CAD build for the part. Positions are in the model's coordinates, mm. A direction names the side the tool comes from. Coordinates: 2 decimals unless noted, no trailing zeros. Loops run counter-clockwise (first coordinate to the right, second up) from the corner with the lowest first, then second, coordinate; pieces in that order, holes last.
1) Wall check: line 1 along Y through (x, z) = (35, -3.05); line 2 along Y through (x, z) = (3.15, -13); line 3 along Y through (x, z) = (44.2, -2.4). Give the ranges that are in metal, low to high.
2) Saw through at D-D, the plane z = -21. Write the cut outline in (x, y).
3) Two-plate mould, pull along Y, no slides. Class faces 3 (the flat face through (14, 0, -7)), 4 (the flat face through (0, 20, -14)), 5 (the cylindrical face through (3, 22, -21)): +Y half, -Y half, draft (parallel to the pull), parting line (faces both ways), or undercut.
4) Saw through at B-B, the plane y = 17. Write the cut outline in (x, z).
5) Saw through at A-A, the plane z = -13. Write the cut outline in (x, y).
6) Pin check, flat tips, straight feed: pin 1 Ø3.5 at (x, y) = (25.8, 8) entering from +Z; pin 2 Ø3 at (x, y) = (42.5, 9.5) entering from -Z. Stop position of each tip, or through.
7) Saw through at C-C, the plane x = 44.2. Write the cut outline in (y, z).
8) Which spindle directions (+Z, -Z, +X, -X, +Y, -Y) get a long thin tool onto all of the face, cutting with end or side? Do faces 1 (the flat face through (9, 35, -9)), 2 (the cylindrical face through (30.24, 24.35, -2.46)). Say none if no direction does.
```python
from build123d import *

# Parameters (mm, degrees)
BOSS_EXTRUDE1_DEPTH = 40
CUT_EXTRUDE1_DEPTH  = 35
BOSS_EXTRUDE2_DEPTH = 5
SKETCH6_R           = 2
CUT_EXTRUDE2_DEPTH  = 70.641941386
SKETCH7_R           = 3.2
SKETCH7_R_2         = 2.1
SKETCH7_R_3         = 2
CUT_EXTRUDE4_DEPTH  = 18.4
SKETCH9_R           = 5.05
CUT_EXTRUDE5_DEPTH  = 3
SKETCH10_R          = 6
CUT_EXTRUDE6_DEPTH  = 73.972597597
SKETCH11_W          = 8
SKETCH11_H          = 40
CUT_EXTRUDE7_DEPTH  = 70.641941386


with BuildPart() as part:
    # Sketch1 → Boss-Extrude1 (new body)
    with BuildSketch(Plane(origin=(0, 0, 0), x_dir=(1, 0, 0), z_dir=(0, 1, 0))):
        Polygon((0, 0), (50, 0), (50, 5), (20, 5), (5, 20), (5, 35), (0, 35), align=None)
    extrude(amount=BOSS_EXTRUDE1_DEPTH)

    # Sketch3 → Cut-Extrude1 (cut)
    with BuildSketch(Plane.XZ):
        Polygon((5, -20), (5, -5), (20, -5), align=None)
    extrude(amount=-CUT_EXTRUDE1_DEPTH, mode=Mode.SUBTRACT)

    # Sketch5 → Boss-Extrude2 (add)
    with BuildSketch(Plane.XZ):
        Polygon((5, -20), (5, -5), (20, -5), align=None)
    extrude(amount=-BOSS_EXTRUDE2_DEPTH)

    # Sketch6 → Cut-Extrude2 (cut, through all)
    with BuildSketch(Plane(origin=(5, 0, 0), x_dir=(0, 0, -1), z_dir=(1, 0, 0))):
        with Locations((13, 30)):
            Circle(SKETCH6_R)
        with Locations((13, 10)):
            Circle(SKETCH6_R)
        with Locations((21, 20)):
            Circle(SKETCH6_R)
    extrude(amount=-CUT_EXTRUDE2_DEPTH, mode=Mode.SUBTRACT)

    # Sketch7 → Cut-Extrude4 (cut)
    with BuildSketch(Plane(origin=(0, 0, -5), x_dir=(-1, 0, 0), z_dir=(0, 0, -1))):
        with Locations((-35, 28)):
            Circle(SKETCH7_R)
        with Locations((-35, 17)):
            Circle(SKETCH7_R_2)
        with Locations((-25.8, 8)):
            Circle(SKETCH7_R_3)
        with Locations((-44.2, 8)):
            Circle(SKETCH7_R_3)
    extrude(amount=-CUT_EXTRUDE4_DEPTH, mode=Mode.SUBTRACT)

    # Sketch9 → Cut-Extrude5 (cut)
    with BuildSketch(Plane.XY):
        with Locations((35, 28)):
            Circle(SKETCH9_R)
    extrude(amount=-CUT_EXTRUDE5_DEPTH, mode=Mode.SUBTRACT)

    # Sketch10 → Cut-Extrude6 (cut, through all)
    with BuildSketch(Plane.XY):
        with Locations((35, 28)):
            Circle(SKETCH10_R)
    extrude(amount=-CUT_EXTRUDE6_DEPTH, mode=Mode.SUBTRACT)

    # Sketch11 → Cut-Extrude7 (cut, through all)
    with BuildSketch(Plane(origin=(5, 0, 0), x_dir=(0, 0, -1), z_dir=(1, 0, 0))):
        with Locations((31, 20)):
            Rectangle(SKETCH11_W, SKETCH11_H)
    extrude(amount=-CUT_EXTRUDE7_DEPTH, mode=Mode.SUBTRACT)


solid = part.part
```
Data:
1. line 1: y = 0 to 14.9, 19.1 to 22, 34 to 40
1. line 2: y = 0 to 8, 12 to 28, 32 to 40
1. line 3: y = 0 to 6, 10 to 40
2. outline: (0, 0) - (5, 0) - (5, 18) - (0, 18) - close; (0, 22) - (5, 22) - (5, 40) - (0, 40) - close
3. face 3: -Y half
3. face 4: draft
3. face 5: undercut
4. outline: (0, -27) - (5, -27) - (5, -5) - (32.9, -5) - (32.9, 0) - (0, 0) - close; (37.1, -5) - (50, -5) - (50, 0) - (37.1, 0) - close
5. outline: (0, 0) - (12, 0) - (12, 5) - (5, 5) - (5, 8) - (0, 8) - close; (0, 12) - (5, 12) - (5, 28) - (0, 28) - close; (0, 32) - (5, 32) - (5, 35) - (12, 35) - (12, 40) - (0, 40) - close
6. pin 1: passes through
6. pin 2: stops at z = -5
7. outline: (0, -5) - (6, -5) - (6, 0) - (0, 0) - close; (10, -5) - (40, -5) - (40, 0) - (10, 0) - close
8. face 1: -Z, +X
8. face 2: +Z, -Z
